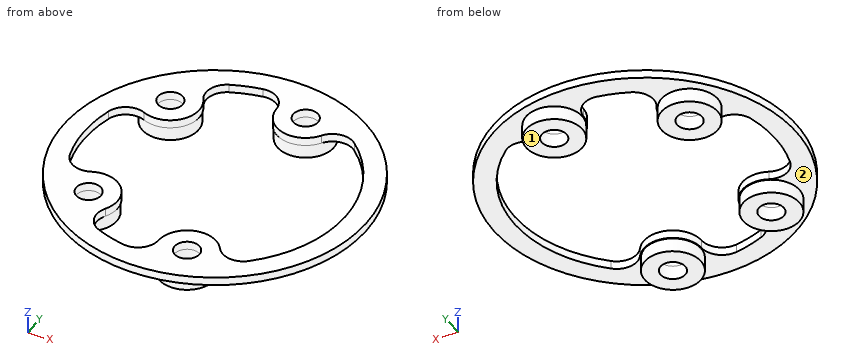
Autodesk Inventor part; units mm, degrees
ref_plane "YZ Plane" through (0, 0, 0) normal (1, 0, 0) x (0, 1, 0)
ref_plane "XZ Plane" through (0, 0, 0) normal (0, 1, 0) x (-1, 0, 0)
ref_plane "XY Plane" through (0, 0, 0) normal (0, 0, 1) x (1, 0, 0)
ref_plane "Work Plane1" through (0, 0, 0) normal (0, 0, 1) x (1, 0, 0)
sketch "Sketch1" plane through (0, 0, 0) normal (0, 0, 1) x (1, 0, 0)
  line L0 (-8.3321, -22.7734) -> (-9.471, -25.3313) construction
  line L1 (-9.471, -25.3313) -> (-12.4875, -23.9883) construction
  line L2 (-12.4875, -23.9883) -> (-11.3486, -21.4303) construction
  line L3 (-11.3486, -21.4303) -> (-8.3321, -22.7734) construction
  line L4 (-16.8745, -17.4155) -> (-18.9553, -19.2891) construction
  line L5 (-18.9553, -19.2891) -> (-21.1648, -16.8352) construction
  line L6 (-21.1648, -16.8352) -> (-19.084, -14.9617) construction
  line L7 (-19.084, -14.9617) -> (-16.8745, -17.4155) construction
  line L8 (-22.4992, -9.0464) -> (-25.1622, -9.9116) construction
  line L9 (-25.1622, -9.9116) -> (-26.1825, -6.7713) construction
  line L10 (-26.1825, -6.7713) -> (-23.5196, -5.906) construction
  line L11 (-23.5196, -5.906) -> (-22.4992, -9.0464) construction
  line L12 (-24.2335, 0.887) -> (-27.0182, 1.1796) construction
  line L13 (-27.0182, 1.1796) -> (-26.6731, 4.4635) construction
  line L14 (-26.6731, 4.4635) -> (-23.8884, 4.1709) construction
  line L15 (-23.8884, 4.1709) -> (-24.2335, 0.887) construction
  line L16 (-21.7777, 10.6669) -> (-24.2026, 12.0669) construction
  line L17 (-24.2026, 12.0669) -> (-22.5516, 14.9266) construction
  line L18 (-22.5516, 14.9266) -> (-20.1267, 13.5266) construction
  line L19 (-20.1267, 13.5266) -> (-21.7777, 10.6669) construction
  line L20 (-15.5563, 18.6025) -> (-17.2021, 20.8678) construction
  line L21 (-17.2021, 20.8678) -> (-14.5307, 22.8086) construction
  line L22 (-14.5307, 22.8086) -> (-12.8849, 20.5434) construction
  line L23 (-12.8849, 20.5434) -> (-15.5563, 18.6025) construction
  line L24 (-6.645, 23.3216) -> (-7.2272, 26.0604) construction
  line L25 (-7.2272, 26.0604) -> (-3.9973, 26.7469) construction
  line L26 (-3.9973, 26.7469) -> (-3.4152, 24.0081) construction
  line L27 (-3.4152, 24.0081) -> (-6.645, 23.3216) construction
  line L28 (3.4152, 24.0081) -> (3.9973, 26.7469) construction
  line L29 (3.9973, 26.7469) -> (7.2272, 26.0604) construction
  line L30 (7.2272, 26.0604) -> (6.645, 23.3216) construction
  line L31 (6.645, 23.3216) -> (3.4152, 24.0081) construction
  line L32 (12.8849, 20.5434) -> (14.5307, 22.8086) construction
  line L33 (14.5307, 22.8086) -> (17.2021, 20.8678) construction
  line L34 (17.2021, 20.8678) -> (15.5563, 18.6025) construction
  line L35 (15.5563, 18.6025) -> (12.8849, 20.5434) construction
  line L36 (20.1267, 13.5266) -> (22.5516, 14.9266) construction
  line L37 (22.5516, 14.9266) -> (24.2026, 12.0669) construction
  line L38 (24.2026, 12.0669) -> (21.7777, 10.6669) construction
  line L39 (21.7777, 10.6669) -> (20.1267, 13.5266) construction
  line L40 (23.8884, 4.1709) -> (26.6731, 4.4635) construction
  line L41 (26.6731, 4.4635) -> (27.0182, 1.1796) construction
  line L42 (27.0182, 1.1796) -> (24.2335, 0.887) construction
  line L43 (24.2335, 0.887) -> (23.8884, 4.1709) construction
  line L44 (23.5196, -5.906) -> (26.1825, -6.7713) construction
  line L45 (26.1825, -6.7713) -> (25.1622, -9.9116) construction
  line L46 (25.1622, -9.9116) -> (22.4992, -9.0464) construction
  line L47 (22.4992, -9.0464) -> (23.5196, -5.906) construction
  line L48 (19.084, -14.9617) -> (21.1648, -16.8352) construction
  line L49 (21.1648, -16.8352) -> (18.9553, -19.2891) construction
  line L50 (18.9553, -19.2891) -> (16.8745, -17.4155) construction
  line L51 (16.8745, -17.4155) -> (19.084, -14.9617) construction
  line L52 (11.3486, -21.4303) -> (12.4875, -23.9883) construction
  line L53 (12.4875, -23.9883) -> (9.471, -25.3313) construction
  line L54 (9.471, -25.3313) -> (8.3321, -22.7734) construction
  line L55 (8.3321, -22.7734) -> (11.3486, -21.4303) construction
  line L56 (1.651, -24.1935) -> (1.651, -26.9935) construction
  line L57 (1.651, -26.9935) -> (-1.651, -26.9935) construction
  line L58 (-1.651, -26.9935) -> (-1.651, -24.1935) construction
  line L59 (-1.651, -24.1935) -> (1.651, -24.1935) construction
  circle A0 centre (0, 0) radius 21.9075 construction
  circle A1 centre (0, 0) radius 29.972 construction
  line L60 (-34.3408, 32.385) -> (-34.3408, -32.385) construction
  line L61 (-34.3408, -32.385) -> (15.5702, -32.385) construction
  line L62 (15.5702, -32.385) -> (15.5702, 32.385) construction
  line L63 (15.5702, 32.385) -> (-34.3408, 32.385) construction
  circle A2 centre (-26.2128, 23.749) radius 1.524 construction
  circle A3 centre (6.9342, -23.749) radius 1.524 construction
  line L64 (-2.9845, -10.0203) -> (-2.9845, -9.271) construction
  line L65 (-2.9845, -9.271) -> (-9.271, -9.271) construction
  line L66 (-9.271, -9.271) -> (-9.271, 9.271) construction
  line L67 (-9.271, 9.271) -> (-2.9845, 9.271) construction
  line L68 (-2.9845, 9.271) -> (-2.9845, 10.0203) construction
  arc A4 (2.9845, 10.0203) -> (-2.9845, 10.0203) centre (0, 10.0203) ccw construction
  line L69 (2.9845, 10.0203) -> (2.9845, 9.271) construction
  line L70 (2.9845, 9.271) -> (9.271, 9.271) construction
  line L71 (9.271, 9.271) -> (9.271, -9.271) construction
  line L72 (9.271, -9.271) -> (2.9845, -9.271) construction
  line L73 (2.9845, -9.271) -> (2.9845, -10.0203) construction
  arc A5 (-2.9845, -10.0203) -> (2.9845, -10.0203) centre (0, -10.0203) ccw construction
  circle A6 centre (4.826, 16.7824) radius 1.905
  circle A7 centre (4.826, -16.7824) radius 1.905
  circle A8 centre (-13.081, 11.5683) radius 1.905
  circle A9 centre (-13.081, -11.5683) radius 1.905
  circle A10 centre (0, 0) radius 23.1775
  arc A11 (1.6885, 19.9311) -> (9.1568, 17.7835) centre (4.826, 16.7824) ccw
  arc A12 (9.1568, -17.7835) -> (1.6885, -19.9311) centre (4.826, -16.7824) ccw
  arc A13 (-12.1243, -15.9092) -> (-17.2723, -10.088) centre (-13.081, -11.5683) ccw
  arc A14 (-17.2723, 10.088) -> (-12.1243, 15.9092) centre (-13.081, 11.5683) ccw
  arc A15 (-12.1243, -15.9092) -> (1.6885, -19.9311) centre (0, 0) ccw
  arc A16 (-17.2723, 10.088) -> (-17.2723, -10.088) centre (0, 0) ccw
  arc A17 (9.1568, -17.7835) -> (9.1568, 17.7835) centre (0, 0) ccw
  arc A18 (1.6885, 19.9311) -> (-12.1243, 15.9092) centre (0, 0) ccw
  dimension "d0" = 2.54
  dimension "d1" = 2.54
  dimension "d2" = 2.54
  dimension "d3" = 2.54
  dimension "d4" = 3.81
  dimension "d5" = 2.54
  dimension "d6" = 3.81
  dimension "d7" = 1.27
  dimension "d9" = 2.54
  dimension "d10" = 3.175
  dimension "d11" = 3.175
  dimension "d12" = 3.175
  dimension "d13" = 3.175
extrude "Extrusion1" add sketch "Sketch1" along normal blind 1.27
fillet "Fillet1" radius 3.175 8 edges at (9.1568, 17.7835, 0.635) (1.6885, 19.9311, 0.635) (-12.1243, 15.9092, 0.635) (-17.2723, 10.088, 0.635) (9.1568, -17.7835, 0.635) (1.6885, -19.9311, 0.635) (-12.1243, -15.9092, 0.635) (-17.2723, -10.088, 0.635)
sketch "Sketch2" plane through (0, 0, 0) normal (0, 0, -1) x (-1, 0, 0)
  circle A0 centre (13.081, -11.5683) radius 1.905
  circle A1 centre (13.081, 11.5683) radius 1.905
  circle A2 centre (-4.826, -16.7824) radius 1.905
  circle A3 centre (-4.826, 16.7824) radius 1.905
  circle A4 centre (-4.826, -16.7824) radius 4.318
  circle A5 centre (-4.826, 16.7824) radius 1.905
  circle A6 centre (-4.826, 16.7824) radius 4.318
  circle A7 centre (13.081, -11.5683) radius 1.905
  circle A8 centre (13.081, -11.5683) radius 4.318
  circle A9 centre (13.081, 11.5683) radius 4.318
  circle A10 centre (0, 0) radius 21.9075 construction
  dimension "d17" = 0.127
extrude "Extrusion2" add sketch "Sketch2" along normal blind 2.159
equation "\"d1\" = d0"
equation "\"d2\" = d1"
equation "\"d3\" = d0"
properties part number "Ring Front"
For this review, take the finished solid that the model builds, in its own axes (mm). Face numbers are marked on the shaded views. A direction names the side the tool comes from. Round coordinates to 2 decimals unless told otherwise and drop trailing zeros. Order: outer loops, then holes, each group sorted by start corner. A loop starts at its lowest first (then second) coordinate and runs counter-clockwise, first axis right, second up. Notation, with made-up numbers: M 1.25,78.5 L 55.25,78.5 A19 cw 55.25,88.5 Z; hole C 10,72 d10. An arc over 180 degrees is marked long. Use a Markdown table: item, result. Add a question column.
Item 1: Add section D-D, the plane x = 4.5. Give the boundary of the cut face in (y, z), then the cut area to 3 significant figures.
Item 2: Add section A-A, the plane y = 0. Give the boundary of the cut face in (x, z), then the cut area to 3 significant figures.
Item 3: To check wall thickness, follow line 1 along X through (y, z) = (-17, -1.7); line 2 along X through (y, z) = (14, 0.1); line 3 along Y through (x, z) = (-13.5, -1.1). State the ranges of each line that lie inside material, in increasing order.
Item 4: Insertion check: pin 1 (1.5 mm diameter, centred on x = 2, z = 0, fed in from +Y); pin 2 (1.5 mm diameter, centred on x = 1.5, z = 0, fed in from +Y). Each pin has a flat end and moves straight along its axis. Give the tip position at first contact, or say it passes through.
Item 5: Add section C-C, the plane x = -12.5. Give the boundary of the cut face in (y, z), then the cut area to 3 significant figures.
Item 6: Tool access review of the marked faces 1 and 2: name each direction out of +Z, -Z, +X, -X, +Y, -Y from which nothing blocks a thin tool from reaching the whole face with its end or side.
Item 7: Add section B-B, the plane z = -1.2. Give the boundary of the cut face in (x, y) (3 decimals).
Geometry results:
| question | item | result |
|---|---|---|
| 1 | outline | M -22.74,0 L -21.09,0 L -21.09,-2.16 L -18.66,-2.16 L -18.66,1.27 L -22.74,1.27 Z; M -14.91,-2.16 L -12.48,-2.16 L -12.48,0 L -12.35,0 L -12.35,1.27 L -14.91,1.27 Z; M 12.35,0 L 12.48,0 L 12.48,-2.16 L 14.91,-2.16 L 14.91,1.27 L 12.35,1.27 Z; M 18.66,-2.16 L 21.09,-2.16 L 21.09,0 L 22.74,0 L 22.74,1.27 L 18.66,1.27 Z |
| 1 | area | 37.8 mm² |
| 2 | outline | M -23.18,0 L -20,0 L -20,1.27 L -23.18,1.27 Z; M 20,0 L 23.18,0 L 23.18,1.27 L 20,1.27 Z |
| 2 | area | 8.06 mm² |
| 3 | line 1 | x = 0.51 to 2.93, 6.72 to 9.14 |
| 3 | line 2 | x = -18.47 to -9.35, 1.36 to 8.29, 14.29 to 18.47 |
| 3 | line 3 | y = -15.87 to -13.43, -9.71 to -7.27, 7.27 to 9.71, 13.43 to 15.87 |
| 4 | pin 1 | stops at y = 23.14 |
| 4 | pin 2 | stops at y = 23.17 |
| 5 | outline | M -19.52,0 L -15.85,0 L -15.85,-2.16 L -13.38,-2.16 L -13.38,1.27 L -19.52,1.27 Z; M -9.75,-2.16 L -7.29,-2.16 L -7.29,0 L -7.16,0 L -7.16,1.27 L -9.75,1.27 Z; M 7.16,0 L 7.29,0 L 7.29,-2.16 L 9.75,-2.16 L 9.75,1.27 L 7.16,1.27 Z; M 13.38,-2.16 L 15.85,-2.16 L 15.85,0 L 19.52,0 L 19.52,1.27 L 13.38,1.27 Z |
| 5 | area | 43.5 mm² |
| 6 | face 1 | -Z, +X, -X, +Y, -Y |
| 6 | face 2 | -Z |
| 7 | outline | C -13.081,-11.568 d8.636; C -13.081,11.568 d8.636; C 4.826,-16.782 d8.636; C 4.826,16.782 d8.636; hole C -13.081,-11.568 d3.81; hole C -13.081,11.568 d3.81; hole C 4.826,-16.782 d3.81; hole C 4.826,16.782 d3.81 |
